```python
from build123d import *

# Parameters (mm, degrees)
SKETCH1_W           = 42.672
SKETCH1_H           = 38.1
BOSS_EXTRUDE1_DEPTH = 4.7625
SKETCH2_R           = 3.25
BOSS_EXTRUDE2_DEPTH = 9.525
SKETCH3_R           = 3.175
CUT_EXTRUDE1_DEPTH  = 9.525
FILLET1_R           = 8


with BuildPart() as part:
    # Sketch1 → Boss-Extrude1 (new body)
    with BuildSketch(Plane(origin=(0, 0, 0), x_dir=(1, 0, 0), z_dir=(0, 1, 0))):
        Rectangle(SKETCH1_W, SKETCH1_H)
    extrude(amount=BOSS_EXTRUDE1_DEPTH)

    # Sketch2 → Boss-Extrude2 (add)
    with BuildSketch(Plane.XY.offset(19.05)):
        with BuildLine():
            Line((-21.336, 4.7625), (-21.336, 27.178))
            ThreePointArc((-21.336, 27.178), (-10.143235589, 38.1), (0.501451896, 26.643181614))
            ThreePointArc((0.501451896, 26.643181614), (6.229357234, 11.237674696), (21.336, 4.7625))
            Line((21.336, 4.7625), (-21.336, 4.7625))
        make_face()
        with Locations((-10.410724966, 27.178)):
            Circle(SKETCH2_R, mode=Mode.SUBTRACT)
    boss_extrude2 = extrude(amount=-BOSS_EXTRUDE2_DEPTH)

    # Mirror1: Boss-Extrude2 across plane
    add(boss_extrude2.mirror(Plane.XY))

    # Sketch3 → Cut-Extrude1 (cut)
    with BuildSketch(Plane(origin=(0, 4.7625, 0), x_dir=(1, 0, 0), z_dir=(0, 1, 0))):
        with Locations(Location((-10.414, 0, 0), (0, 0, 270))):
            Circle(SKETCH3_R)
        with Locations(Location((11.684, 0, 0), (0, 0, 270))):
            Circle(SKETCH3_R)
    extrude(amount=-CUT_EXTRUDE1_DEPTH, mode=Mode.SUBTRACT)

    # Fillet1
    fillet1_edges = [part.edges().sort_by_distance(p)[0] for p in [
        (21.336, 2.38125, -19.05),
        (21.336, 2.38125, 19.05),
    ]]
    fillet(fillet1_edges, radius=FILLET1_R)


solid = part.part
```
The model under review builds one solid part; all positions refer to its coordinate system, in mm. A direction names the side the tool comes from. Round coordinates to 2 decimals unless told otherwise and drop trailing zeros. Order: outer loops, then holes, each group sorted by start corner. A loop starts at its lowest first (then second) coordinate and runs counter-clockwise, first axis right, second up.
(1) Take a section at A-A, the plane z = 0. State the section outline as (x, y) points, plus the area to 3 significant figures.
Working result:
outline: (-21.34, 0) - (-13.59, 0) - (-13.59, 4.76) - (-21.34, 4.76) - close; (-7.24, 0) - (8.51, 0) - (8.51, 4.76) - (-7.24, 4.76) - close; (14.86, 0) - (21.34, 0) - (21.34, 4.76) - (14.86, 4.76) - close
area: 143 mm2
(2) For P1, Ø3, axis at x = 10, z = -13.5, coming from the +Y side; P2, Ø5, axis at x = -10.41, y = 27.18, coming from the -Z side; P3, Ø1.5, axis at x = 0.5, z = 3.5, coming from the +Y side; P4, Ø9.5, axis at x = -8, z = 5, coming from the +Y side, all flat-tipped, find the tip position at first contact; note any pin that passes through.
Working result:
P1: stops at y = 9.18
P2: passes through
P3: stops at y = 4.76
P4: stops at y = 38.06
(3) Tool access review of faces 1 (the face through (-9, 18, -9.525)), 2 (the face through (-8, 15, -19.05)): name each direction out of +Z, -Z, +X, -X, +Y, -Y from which nothing blocks a thin tool from reaching the whole face with its end or side.
Working result:
face 1: +X, -X, +Y
face 2: -Z, +X, -X, +Y, -Y
(4) Take a section at D-D, the plane z = 16. State the section outline as (x, y) points, plus the area to 3 significant figures.
Working result:
outline: (-21.34, 0) - (19.62, 0) - (19.62, 4.83) arc R20.86 cw to (0.5, 26.64) arc R10.93 ccw (long way) to (-21.34, 27.18) - close; hole circle Ø6.5 at (-10.41, 27.18)
area: 932 mm2
(5) Take a section at B-B, the plane y = 13.5. State the section outline as (x, z) points (3 decimals).
Working result:
outline: (-21.336, -19.05) - (4.36, -19.05) - (4.36, -9.525) - (-21.336, -9.525) - close; (-21.336, 9.525) - (4.36, 9.525) - (4.36, 19.05) - (-21.336, 19.05) - close
(6) Wall thickness on L1, parallel to X at y = 3, z = 0; L2, parallel to Z at x = -1, y = 18 (3 decimals); L3, parallel to X at y = 3, z = -2.5: over which ranges is each line inside the solid? List them lowest first.
Working result:
L1: x = -21.34 to -13.59, -7.24 to 8.51, 14.86 to 21.34
L2: z = -19.05 to -9.525, 9.525 to 19.05
L3: x = -21.34 to -12.37, -8.46 to 9.73, 13.64 to 21.34
(7) Mouldability with a two-part tool opening along Y and no side actions: class faces 3 (the face through (14.36, 2.41, 1.71)), 4 (the face through (0, 0, 0)), 5 (the face through (-10.83, 30.4, 14.35)), 6 (the face through (0, 4.762, 0)) as released by +Y, released by -Y, zero draft, split by the parting line, or undercut.
Working result:
face 3: zero draft
face 4: released by -Y
face 5: undercut
face 6: released by +Y
